Can you work these out from the model? Positions are in its coordinate system, mm. A direction names the side the tool comes from. Give positions to 0.01 mm unless a question says otherwise; leave off trailing zeros. Order: outer loops, then holes, each group sorted by start corner. A loop starts at its lowest first (then second) coordinate and runs counter-clockwise, first axis right, second up. Notation, with made-up numbers: M -12.5,-17 L 22.5,-17 A18 cw 22.5,-7 Z; hole C 51.25,52.5 d5. An arc over 180 degrees is marked long. One line per question, with ' | ' between items. Start each with the question number.
1) I'm going to push flat-ended pins straight in: pin 1 Ø3 at (y, z) = (1, -10) entering from -X; pin 2 Ø1.8 at (x, y) = (-32.5, 6.5) entering from -Z; pin 3 Ø2 at (x, y) = (-16.5, 2) entering from +Z. Where does each tip first touch, or does it pass through?
2) Please list where these lines run through material, in increasing order: line 1 along Z through (x, y) = (-36, 7.75); line 2 along X through (y, z) = (6.25, -123.5); line 3 along X through (y, z) = (7.25, -160). Write a range as [from, to].
3) If we section it at C-C, the plane z = -92.5: Please give me the cut outline in (x, y).
4) If we section it at B-B, the plane z = -27.5: Please give me the cut outline in (x, y).
5) Thinking about a two-plate mould opening in X: for faces 4 (the flat face through (-32, 5, -20.11)), 5 (the cylindrical face through (-1.141, 1.203, -87.914)), 6 (the cylindrical face through (-12.941, 1.203, -1.141)), which applies, +X half, -X half, draft (parallel to the pull), parting line (faces both ways), or undercut?
6) For faces 1 (the flat face through (-49, 7, -106.66)), 2 (the flat face through (-48.808, 2, -146)), 3 (the flat face through (-10.261, 4.764, -21.691)), which set-ups out of +Z, -Z, +X, -X, +Y, -Y let a thin tool reach every point of the face, with its end or its side?
7) If we section it at A-A, the plane z = -134: Please give me the cut outline in (x, y).
Autodesk Inventor part; units mm, degrees
ref_plane "Work Plane1" through (-38.25, 4, -70.11) normal (0, -1, 0) x (1, 0, 0)
ref_plane "YZ Plane" through (0, 0, 0) normal (1, 0, 0) x (0, 1, 0)
ref_plane "XZ Plane" through (0, 0, 0) normal (0, 1, 0) x (-1, 0, 0)
sketch "Sketch1" plane through (0, 0, 0) normal (0, 1, 0) x (-1, 0, 0)
  line L0 (0, 0) -> (0, -173.4)
  line L1 (0, -173.4) -> (62.5, -173.4)
  line L2 (62.5, -173.4) -> (62.5, 0)
  line L3 (62.5, 0) -> (0, 0)
  dimension "d0" = 173.4
  dimension "d1" = 62.5
extrude "Extrusion1" add sketch "Sketch1" along normal blind 10
sketch "Sketch2" plane through (0, 10, 0) normal (0, 1, 0) x (1, 0, 0)
  line L0 (0, 0) -> (0, 102.12)
  line L1 (0, 0) -> (0, 173.4)
  line L2 (0, 102.12) -> (-62.5, 102.12)
  line L3 (-62.5, 173.4) -> (-62.5, 0)
  line L4 (-31.25, 102.12) -> (-31.25, 0)
  line L5 (-62.5, 0) -> (0, 0)
  line L6 (-31.25, 102.12) -> (-37.45, 102.12)
  line L7 (-37.45, 102.12) -> (-31.25, 102.12)
  line L8 (-31.25, 102.12) -> (-25.05, 102.12)
  line L9 (-25.05, 102.12) -> (-31.25, 102.12)
  line L10 (-31.25, 102.12) -> (-31.25, 85.22)
  line L11 (-31.25, 85.22) -> (-25.05, 85.22)
  line L12 (-25.05, 85.22) -> (-25.05, 102.12)
  line L13 (-31.25, 85.22) -> (-37.45, 85.22)
  line L14 (-37.45, 85.22) -> (-37.45, 102.12)
  line L15 (-31.25, 102.12) -> (-31.25, 108.42)
  line L16 (-31.25, 108.42) -> (-25.05, 108.42)
  line L17 (-25.05, 108.42) -> (-25.05, 102.12)
  line L18 (-37.45, 102.12) -> (-37.45, 108.42)
  line L19 (-37.45, 108.42) -> (-31.25, 108.42)
  line L20 (-31.25, 108.42) -> (-31.25, 173.4)
  line L21 (0, 173.4) -> (-62.5, 173.4)
  line L22 (-31.25, 140.91) -> (-31.25, 120.66)
  line L23 (-31.25, 120.66) -> (-22.25, 120.66)
  line L24 (-22.25, 120.66) -> (-22.25, 165.66)
  line L25 (-22.25, 165.66) -> (-40.25, 165.66)
  line L26 (-40.25, 165.66) -> (-40.25, 120.66)
  line L27 (-40.25, 120.66) -> (-31.25, 120.66)
  line L28 (-40.25, 120.66) -> (-40.25, 126.66)
  line L29 (-40.25, 126.66) -> (-44.25, 126.66)
  line L30 (-44.25, 126.66) -> (-47.25, 126.66)
  line L31 (-47.25, 126.66) -> (-47.25, 106.66)
  line L32 (-47.25, 106.66) -> (-50.25, 106.66)
  line L33 (-50.25, 106.66) -> (-50.25, 126.66)
  line L34 (-50.25, 126.66) -> (-47.25, 126.66)
  line L35 (-31.25, 0) -> (-31.25, 85.22)
  line L36 (-31.25, 42.61) -> (-31.25, 20.11)
  line L37 (-31.25, 20.11) -> (-31.25, 42.61)
  line L38 (-31.25, 42.61) -> (-31.25, 65.11)
  line L39 (-31.25, 65.11) -> (-53.75, 65.11)
  line L40 (-53.75, 65.11) -> (-53.75, 20.11)
  line L41 (-53.75, 20.11) -> (-8.75, 20.11)
  line L42 (-8.75, 20.11) -> (-8.75, 65.11)
  line L43 (-8.75, 65.11) -> (-31.25, 65.11)
  line L44 (-22.25, 120.66) -> (-40.25, 120.66)
  line L45 (-40.25, 120.66) -> (-40.25, 165.66)
  line L46 (-40.25, 165.66) -> (-22.25, 165.66)
  line L47 (-22.25, 165.66) -> (-22.25, 120.66)
  line L48 (-53.75, 65.11) -> (-48.75, 65.11)
  line L49 (-48.75, 65.11) -> (-8.75, 65.11)
  line L50 (-8.75, 65.11) -> (-13.75, 65.11)
  line L51 (-13.75, 65.11) -> (-13.75, 70.11)
  line L52 (-13.75, 70.11) -> (-48.75, 70.11)
  line L53 (-48.75, 70.11) -> (-48.75, 65.11)
  line L54 (-48.75, 65.11) -> (-13.75, 65.11) construction
  line L55 (-18.75, 70.11) -> (-43.75, 70.11)
  arc A0 (-43.75, 70.11) -> (-48.75, 65.11) centre (-43.75, 65.11) ccw
  arc A1 (-13.75, 65.11) -> (-18.75, 70.11) centre (-18.75, 65.11) ccw
  line L56 (-8.75, 65.11) -> (-8.75, 55.11)
  line L57 (-8.75, 55.11) -> (-8.75, 45.11)
  line L58 (-8.75, 45.11) -> (-53.75, 45.11)
  line L59 (-53.75, 45.11) -> (-53.75, 55.11)
  line L60 (-53.75, 45.11) -> (-53.75, 55.11) construction
  line L61 (-51.25, 47.61) -> (-51.25, 52.61)
  line L62 (-56.25, 52.61) -> (-56.25, 47.61)
  arc A2 (-56.25, 47.61) -> (-51.25, 47.61) centre (-53.75, 47.61) ccw
  arc A3 (-51.25, 52.61) -> (-56.25, 52.61) centre (-53.75, 52.61) ccw
  line L63 (-8.75, 45.11) -> (-8.75, 55.11) construction
  line L64 (-6.25, 47.61) -> (-6.25, 52.61)
  line L65 (-11.25, 52.61) -> (-11.25, 47.61)
  arc A4 (-11.25, 47.61) -> (-6.25, 47.61) centre (-8.75, 47.61) ccw
  arc A5 (-6.25, 52.61) -> (-11.25, 52.61) centre (-8.75, 52.61) ccw
  line L66 (-40.25, 165.66) -> (-40.25, 173.4)
  line L67 (-22.25, 165.66) -> (-22.25, 173.4)
  line L68 (-40.25, 173.4) -> (-22.25, 173.4) construction
  line L69 (-37.75, 170.9) -> (-24.75, 170.9)
  line L70 (-24.75, 175.9) -> (-37.75, 175.9)
  arc A6 (-37.75, 175.9) -> (-37.75, 170.9) centre (-37.75, 173.4) ccw
  arc A7 (-24.75, 170.9) -> (-24.75, 175.9) centre (-24.75, 173.4) ccw
  line L71 (-31.25, 102.12) -> (-34.35, 102.12)
  line L72 (-28.15, 102.12) -> (-31.25, 102.12)
  line L73 (-34.35, 102.12) -> (-28.15, 102.12) construction
  line L74 (-32.35, 100.12) -> (-30.15, 100.12)
  line L75 (-30.15, 104.12) -> (-32.35, 104.12)
  arc A8 (-32.35, 104.12) -> (-32.35, 100.12) centre (-32.35, 102.12) ccw
  arc A9 (-30.15, 100.12) -> (-30.15, 104.12) centre (-30.15, 102.12) ccw
  arc A10 (-32.35, 110.42) -> (-32.35, 106.42) centre (-32.35, 108.42) ccw
  arc A11 (-30.15, 106.42) -> (-30.15, 110.42) centre (-30.15, 108.42) ccw
  line L76 (-32.35, 110.42) -> (-30.15, 110.42)
  point P0 (-31.25, 165.66)
  point P1 (-31.25, 165.66)
  point P2 (-53.75, 50.11)
  point P3 (-8.75, 50.11)
  point P4 (-34.35, 108.42)
  point P5 (-28.15, 108.42)
  dimension "d4" = 102.12
  dimension "d5" = 6.2
  dimension "d6" = 6.2
  dimension "d7" = 16.9
  dimension "d8" = 6.3
  dimension "d11" = 20.25
  dimension "d12" = 9
  dimension "d13" = 45
  dimension "d14" = 18
  dimension "d15" = 6
  dimension "d16" = 4
  dimension "d17" = 3
  dimension "d18" = 20
  dimension "d19" = 3
  dimension "d20" = 22.5
  dimension "d21" = 22.5
  dimension "d22" = 22.5
  dimension "d23" = 45
  dimension "d24" = 5
  dimension "d25" = 5
  dimension "d26" = 5
  dimension "d27" = 10
  dimension "d28" = 10
  dimension "d29" = 5
  dimension "d30" = 5
  dimension "d36" = 5
  dimension "d37" = 4
  dimension "d39" = 4
extrude "Extrusion2" cut sketch "Sketch2" against normal through all contours L12 L11 L4 L74 A9 L2 | L2 A9 L75 L15 L16 L17 | L41 L40 L58 L4 | L4 L58 L42 L41 | A7 L69 L20 L21 | A9 L74 L4 L2 | L2 L15 L75 A9 | L31 L32 L33 L34 | L20 L69 A6 L21 | L24 L23 L20 L25 | L4 L74 A8 L2 | L2 A8 L75 L15 | L13 L14 L2 A8 L74 L4 | L16 L20 L76 A11 | L58 A2 L61 A3 L40 L39 L4 | L4 L43 L42 A5 L65 A4 L58 | A2 L62 A3 L40 | L40 A3 L61 A2 | A4 L65 A5 L42 | L42 A5 L64 A4 | L18 L19 L15 L75 A8 L2 | L20 L27 L26 L25 | L52 A1 L43 L4 | L4 L39 A0 L52 | L19 A10 L76 L20
sketch "Sketch3" plane through (0, 10, 0) normal (0, 1, 0) x (1, 0, 0)
  point P0 (0, 0)
sketch "Sketch4" plane through (0, 0, 0) normal (0, -1, 0) x (1, 0, 0)
  line L0 (-8.75, -20.11) -> (-53.75, -20.11)
  line L1 (-53.75, -20.11) -> (-8.75, -20.11)
  line L2 (-8.75, -20.11) -> (-31.25, -20.11)
  line L3 (-62.5, 0) -> (0, 0)
  line L4 (-31.25, 0) -> (-31.25, -20.11)
  line L5 (-31.25, -20.11) -> (-26.25, -20.11)
  line L6 (-26.25, -20.11) -> (-36.25, -20.11)
  line L7 (-36.25, -20.11) -> (-36.25, 0)
  line L8 (-36.25, 0) -> (-26.25, 0)
  line L9 (-26.25, 0) -> (-26.25, -20.11)
  line L10 (-40.25, -165.66) -> (-40.25, -120.66)
  line L11 (-40.25, -120.66) -> (-47.25, -120.66)
  line L12 (-47.25, -126.66) -> (-47.25, -106.66)
  line L13 (-48.8082, -126.9328) -> (-40.25, -126.9328)
  line L14 (-40.25, -126.9328) -> (-48.8082, -126.9328)
  line L15 (-40.25, -165.66) -> (-22.25, -165.66)
  line L16 (-40.25, -165.66) -> (-48.8082, -165.66)
  line L17 (-48.8082, -165.66) -> (-48.8082, -126.9328)
  line L18 (-22.25, -120.66) -> (-22.25, -165.66)
  line L19 (-22.25, -165.66) -> (-15.25, -165.66)
  line L20 (-15.25, -165.66) -> (-15.25, -120.66)
  line L21 (-15.25, -120.66) -> (-22.25, -120.66)
  line L22 (-40.25, -120.66) -> (-22.25, -120.66)
  line L23 (-22.25, -120.66) -> (-40.25, -120.66)
  line L24 (-40.25, -120.66) -> (-40.25, -126.9328)
  line L25 (-40.25, -165.66) -> (-40.25, -126.9328)
  line L26 (-22.25, -120.66) -> (-22.25, -165.66)
  line L27 (-40.25, -165.66) -> (-40.25, -173.4)
  line L28 (0, -173.4) -> (-62.5, -173.4)
  line L29 (-48.8082, -165.66) -> (-40.25, -173.4)
  line L30 (-22.25, -165.66) -> (-22.25, -173.4)
  line L31 (-22.25, -173.4) -> (-15.25, -165.66)
  line L32 (-40.25, -173.4) -> (-22.25, -173.4)
  line L33 (-37.45, -108.42) -> (-37.45, -85.22)
  line L34 (-25.05, -85.22) -> (-25.05, -108.42)
  line L35 (-37.45, -108.42) -> (-25.05, -108.42)
  line L36 (-25.05, -108.42) -> (-22.25, -120.66)
  line L37 (-37.45, -108.42) -> (-40.25, -120.66)
  line L38 (-43.75, -70.11) -> (-18.75, -70.11)
  line L39 (-50.25, -126.66) -> (-50.25, -106.66)
  line L40 (-43.75, -70.11) -> (-50.25, -106.66)
  line L41 (-47.25, -106.66) -> (-50.25, -106.66)
  line L42 (-47.25, -106.66) -> (-40.25, -70.11)
  line L43 (-18.75, -70.11) -> (-15.25, -120.66)
  line L44 (-25.05, -108.42) -> (-37.45, -108.42)
  line L45 (-25.05, -85.22) -> (-37.45, -85.22)
  line L46 (-25.05, -108.42) -> (-25.05, -85.22)
  line L47 (-25.05, -85.22) -> (-43.1438, -85.22)
  line L48 (-37.45, -108.42) -> (-47.25, -120.66)
  line L49 (-48.8082, -126.9328) -> (-48.8082, -120.66)
  line L50 (-48.8082, -120.66) -> (-47.25, -120.66)
  line L51 (-37.45, -108.42) -> (-47.25, -108.42)
  line L52 (-37.45, -108.42) -> (-38.0612, -111.0919)
  line L53 (-38.0612, -111.0919) -> (-47.25, -111.0919)
  point P0 (-39.5893, -111.0919)
  dimension "d31" = 5
  dimension "d32" = 10
  dimension "d33" = 7
extrude "Extrusion3" cut sketch "Sketch4" against normal blind 4 contours L0 L4 L3 L9 | L0 L7 L3 L4 | L16 L17 L13 L10 | L27 L29 L16 | L15 L30 L28 L27 | L13 L49 L50 L11 L10 | L18 L21 L20 L19 | L19 L31 L30 | L37 L35 L36 L22 | L11 L48 L53 L37 | L36 L34 L45 L47 L42 L38 L43 L21 | L53 L48 L37 | L12 L51 L48 L53 | L42 L41 L40 L38
sketch "Sketch5" plane through (-40.25, 10, -165.66) normal (0, 0, 1) x (1, 0, 0)
  point P0 (40.25, -10)
fillet "Fillet1" radius 4 6 edges at (0, 0, -86.7) (-62.5, 0, -86.7) (-49.375, 0, 0) (-13.125, 0, 0) (-51.375, 0, -173.4) (-11.125, 0, -173.4)
ref_plane "Work Plane1" through (-38.25, 4, -70.11) normal (0, -1, 0) x (1, 0, 0)
sketch "Sketch6" plane through (-38.25, 4, -70.11) normal (0, -1, 0) x (1, 0, 0)
  line L0 (-15.5, 15) -> (-15.5, 5)
  arc A0 (-10.5, 5) -> (-5.5, 0) centre (-5.5, 5) ccw
  line L1 (-15.5, 5) -> (-10.5, 5)
  line L2 (-15.5, 5) -> (-10.5, 5)
  line L3 (-10.5, 5) -> (-15.5, 5)
  line L4 (-15.5, 5) -> (-15.5, 10)
  line L5 (-15.5, 10) -> (-10.5, 5)
  line L6 (-15.5, 50) -> (-15.5, 25)
  line L7 (-15.5, 50) -> (-15.5, 45)
  line L8 (-15.5, 45) -> (-15.5, 50)
  line L9 (-15.5, 50) -> (2, 50)
  line L10 (-15.5, 50) -> (-10.5, 50)
  line L11 (-10.5, 50) -> (-15.5, 45)
  line L12 (-5.5, 0) -> (19.5, 0)
  line L13 (7, 0) -> (7, 50)
  line L14 (12, 50) -> (2, 50)
  line L15 (29.5, 15) -> (29.5, 5)
  line L16 (29.5, 5) -> (24.5, 5)
  line L17 (29.5, 10) -> (24.5, 5)
  line L18 (29.5, 50) -> (29.5, 45)
  line L19 (29.5, 50) -> (12, 50)
  line L20 (24.5, 50) -> (29.5, 45)
  line L21 (-2, -50.55) -> (-2, -95.55)
  line L22 (-2, -50.55) -> (-2, -53.05)
  line L23 (-2, -53.05) -> (-2, -50.55)
  line L24 (-2, -50.55) -> (-2, -53.05)
  line L25 (-2, -53.05) -> (0.5, -53.05)
  line L26 (0.5, -53.05) -> (0.5, -50.55)
  line L27 (16, -50.55) -> (-2, -50.55)
  line L28 (-2, -50.55) -> (0.5, -50.55)
  line L29 (-2, -50.55) -> (-2, -53.05)
  line L30 (7, -50.55) -> (7, -95.55)
  line L31 (-2, -95.55) -> (16, -95.55)
  line L32 (-2, -95.55) -> (-2, -93.05)
  line L33 (-2, -93.05) -> (0.5, -93.05)
  line L34 (0.5, -93.05) -> (0.5, -95.55)
  line L35 (0.5, -95.55) -> (-2, -95.55)
  line L36 (16, -50.55) -> (16, -95.55)
  line L37 (16, -50.55) -> (16, -53.05)
  line L38 (16, -53.05) -> (13.5, -53.05)
  line L39 (13.5, -53.05) -> (13.5, -50.55)
  line L40 (-2, -50.55) -> (16, -50.55)
  line L41 (16, -95.55) -> (-2, -95.55)
  line L42 (16, -93.05) -> (13.5, -93.05)
  line L43 (13.5, -93.05) -> (13.5, -95.55)
  point P0 (38.25, 70.11)
  dimension "d40" = 5
  dimension "d41" = 5
  dimension "d42" = 5
  dimension "d43" = 2.5
  dimension "d44" = 2.5
  dimension "d45" = 2.5
  dimension "d46" = 2.5
extrude "Extrusion4" add sketch "Sketch6" against normal blind 2 contours L5 L1 L0 | L11 L6 L9 | L19 L18 L20 | L15 L16 L17 | L27 L26 L25 L21 | L33 L34 L31 L21 | L27 L36 L38 L39 | L43 L42 L36 L31
chamfer "Chamfer1" distance 3.535 distance2 2 1 edges at (-51.25, 6, -22.61) measured on face at (-52.0833, 6, -21.7767)
chamfer "Chamfer2" distance 3.535 distance2 2 1 edges at (-51.25, 6, -62.61) measured on face at (-52.0833, 6, -63.4433)
chamfer "Chamfer3" distance 3.535 distance2 2 1 edges at (-11.25, 6, -62.61) measured on face at (-10.4167, 6, -63.4433)
chamfer "Chamfer4" distance 3.535 distance2 2 1 edges at (-11.25, 6, -22.61) measured on face at (-10.4167, 6, -21.7767)
chamfer "Chamfer5" distance 2.5 distance2 2 1 edges at (-23.5, 6, -123.16) measured on face at (-23.0833, 6, -122.3267)
chamfer "Chamfer6" distance 2.5 distance2 2 1 edges at (-39, 6, -123.16) measured on face at (-39.4167, 6, -121.4933)
chamfer "Chamfer7" distance 2.5 distance2 2 1 edges at (-39, 6, -163.16) measured on face at (-39.4167, 6, -163.9933)
chamfer "Chamfer8" distance 2.5 distance2 2 1 edges at (-23.5, 6, -163.16) measured on face at (-23.9167, 6, -163.9933)
properties part number "inside"
Results found:
1) pin 1: stops at x = -62.21 | pin 2: stops at z = -170.9 | pin 3: stops at z = -0.13
2) line 1: z = [-170.9, -165.66], [-120.66, -108.42], [-85.22, -70.11], [-20.11, 0] | line 2: x = [-62.5, -50.25], [-47.25, -40.25], [-22.25, 0] | line 3: x = [-62.5, -40.25], [-22.25, 0]
3) outline: M -62.5,4 A4 ccw -58.5,0 L -47.73,0 L -47.73,4 L -44.54,4 L -44.54,0 L -37.45,0 L -37.45,10 L -62.5,10 Z; M -25.05,4 L -17.2,4 L -17.2,0 L -4,0 A4 ccw 0,4 L 0,10 L -25.05,10 Z
4) outline: M -62.5,4 A4 ccw -58.5,0 L -53.75,0 L -53.75,10 L -62.5,10 Z; M -8.75,0 L -4,0 A4 ccw 0,4 L 0,10 L -8.75,10 Z
5) face 4: undercut | face 5: +X half | face 6: draft
6) face 1: +Y, -Y | face 2: -Y | face 3: +Y
7) outline: M -62.5,4 A4 ccw -58.5,0 L -48.81,0 L -48.81,4 L -40.25,4 L -40.25,10 L -62.5,10 Z; M -22.25,4 L -15.25,4 L -15.25,0 L -4,0 A4 ccw 0,4 L 0,10 L -22.25,10 Z
